from build123d import *

# Parameters (mm, degrees)
CROQUIS1_W              = 97
CROQUIS1_H              = 87
SALIENTE_EXTRUIR1_DEPTH = 69
CROQUIS2_R              = 40.625765917
CORTAR_EXTRUIR1_DEPTH   = 0.1
CROQUIS3_W              = 9.671731422
CROQUIS3_H              = 3.578358675
CORTAR_EXTRUIR2_DEPTH   = 2


with BuildPart() as part:
    # Croquis1 → Saliente-Extruir1 (new body)
    with BuildSketch(Plane(origin=(0, 0, 0), x_dir=(1, 0, 0), z_dir=(0, 1, 0))):
        Rectangle(CROQUIS1_W, CROQUIS1_H)
    extrude(amount=SALIENTE_EXTRUIR1_DEPTH)

    # Croquis2 → Cortar-Extruir1 (cut)
    with BuildSketch(Plane(origin=(0, 69, 0), x_dir=(1, 0, 0), z_dir=(0, 1, 0))):
        Circle(CROQUIS2_R)
    extrude(amount=-CORTAR_EXTRUIR1_DEPTH, mode=Mode.SUBTRACT)

    # Croquis3 → Cortar-Extruir2 (cut)
    with BuildSketch(Plane(origin=(48.5, 0, 0), x_dir=(0, 0, -1), z_dir=(1, 0, 0))):
        with Locations((4.835865711, 1.789179338)):
            Rectangle(CROQUIS3_W, CROQUIS3_H)
    extrude(amount=-CORTAR_EXTRUIR2_DEPTH, mode=Mode.SUBTRACT)


solid = part.part
Read the model definition and answer for the solid it produces. Units are mm, in the model's axes. A direction names the side the tool comes from. Round coordinates to 2 decimals unless told otherwise and drop trailing zeros. Use one line per item in the form item = value. Start each with the question number.
(1) Flat-ended cylindrical pins translate along their axes: pin 1 Ø1.6 at (x, z) = (47, -3.5) entering from -Y; pin 2 Ø24.5 at (x, z) = (1.5, 7) entering from +Y. Find the tip coordinate at first contact, or state that the pin passes through.
(2) Find the intervals of material crossed by line 1 along Y through (x, z) = (9, 31), in increasing order. Write a range as from..to.
(3) Determine the mould class of faces 3 (the face through (-1, 68.9, -1)), 4 (the face through (-1, 34, 43.5)), 5 (the face through (-11.5, 69, -39.3)) for opening direction Z: +Z half, -Z half, draft (parallel to the pull), parting line (faces both ways), or undercut.
(4) For faces 1 (the face through (48.5, 34, 1)), 2 (the face through (46.5, 2, -5)), determine the directions among +Z, -Z, +X, -X, +Y, -Y from which every point of the face is accessible in a straight line to the end or side of a thin tool.
Checked values:
q1.pin_1 = 0
q1.pin_2 = 68.9
q2.line_1 = 0..68.9
q3.face_3 = undercut
q3.face_4 = +Z half
q3.face_5 = draft
q4.face_1 = +Z, -Z, +X, +Y, -Y
q4.face_2 = +X, -Y
